Here's how the part is built. I have some questions about the finished solid (model axes, mm). A direction names the side the tool comes from. Round coordinates to 2 decimals unless told otherwise and drop trailing zeros. Write each loop counter-clockwise with the first axis right and the second up, starting at its lowest first coordinate (ties: lowest second). Pieces come first, ordered by that corner, then holes. Notation, with made-up numbers: (24.5, 30) -> (33.5, 30) arc R25 ccw to (33.5, 56) -> close; hole circle Ø4 at (16.5, -28). An arc over 180 degrees is marked (long way). Answer as CSV lines item,"result".
from build123d import *

# Parameters (mm, degrees)
F2_DEPTH  = 6.35
F3_DEPTH  = 25.4
F5_DEPTH  = 63.5
F6_W      = 35.5600007778
F6_H      = 6.6786579132
F7_DEPTH  = 25.4
F8_W      = 6.5081897405
F8_H      = 35.5600007778
F9_DEPTH  = 57.15
F10_W     = 35.5600007778
F10_H     = 6.35
F11_DEPTH = 19.05
F12_R     = 5.08
F13_R     = 5.08
F14_R     = 5.08
F15_R     = 5.08
F16_R     = 5.08


# Not quite as in the source:
# - two fillets or chamfers of one size are made in one step


with BuildPart() as f2:
    # F0 (on Top) → F2 (new body)
    with BuildSketch(Plane.XY):
        with BuildLine():
            ThreePointArc((-18.3481574059, -1.8204556262), (-18.2829820174, -0.6015784588), (-18.3481574059, 0.6172987085))
            Line((-18.3481574059, 0.6172987085), (-18.3481574059, -1.8204556262))
        make_face()
        with BuildLine():
            Line((-29.7129820174, 10.8284215412), (-64.0681574059, 10.8284215412))
            Line((-64.0681574059, 10.8284215412), (-64.0681574059, 5.8474093676))
            Line((-64.0681574059, 5.8474093676), (-65.235733552, 5.8474093676))
            Line((-65.235733552, 5.8474093676), (-65.235733552, -6.7013129592))
            Line((-65.235733552, -6.7013129592), (-64.0681574059, -6.7013129592))
            Line((-64.0681574059, -6.7013129592), (-64.0681574059, -12.0315784588))
            Line((-64.0681574059, -12.0315784588), (-60.0158534944, -12.0315784588))
            Line((-60.0158534944, -12.0315784588), (-60.0158534944, -14.5130921155))
            Line((-60.0158534944, -14.5130921155), (-49.2716534944, -14.5130921155))
            Line((-49.2716534944, -14.5130921155), (-49.2716534944, -12.0315784588))
            Line((-49.2716534944, -12.0315784588), (-29.7129820174, -12.0315784588))
            ThreePointArc((-29.7129820174, -12.0315784588), (-22.0738350108, -9.1038330429), (-18.3481574059, -1.8204556262))
            Line((-18.3481574059, -1.8204556262), (-18.3481574059, 0.6172987085))
            ThreePointArc((-18.3481574059, 0.6172987085), (-22.0738350108, 7.9006761252), (-29.7129820174, 10.8284215412))
        make_face()
    extrude(amount=-F2_DEPTH)

    # F1 (on Top) → F3 (join)
    with BuildSketch(Plane.XY):
        with BuildLine():
            Line((-42.9216531055, -18.3815788478), (-29.7129820174, -18.3815788478))
            ThreePointArc((-29.7129820174, -18.3815788478), (-17.6903920931, -13.7006526758), (-11.9981570169, -2.1225613757))
            Line((-11.9981570169, -2.1225613757), (-11.9981570169, 0.919404458))
            ThreePointArc((-11.9981570169, 0.919404458), (-17.6903920931, 12.4974957581), (-29.7129820174, 17.1784219301))
            Line((-29.7129820174, 17.1784219301), (-70.4181577948, 17.1784219301))
            Line((-70.4181577948, 17.1784219301), (-70.4181577948, 12.1974097565))
            Line((-70.4181577948, 12.1974097565), (-70.4181577948, -13.0513133481))
            Line((-70.4181577948, -13.0513133481), (-70.4181577948, -18.3815788478))
            Line((-70.4181577948, -18.3815788478), (-66.3658538833, -18.3815788478))
            Line((-66.3658538833, -18.3815788478), (-42.9216531055, -18.3815788478))
        make_face()
    extrude(amount=-F3_DEPTH)

    # F4 (on face) → F5 (join)
    with BuildSketch(Plane.XY):
        with BuildLine():
            Line((-42.9216538833, -18.3815788478), (-29.7129820174, -18.3815788478))
            ThreePointArc((-29.7129820174, -18.3815788478), (-17.6903920931, -13.7006526758), (-11.9981570169, -2.1225613757))
            Line((-11.9981570169, -2.1225613757), (-11.9981570169, 0.919404458))
            ThreePointArc((-11.9981570169, 0.919404458), (-17.6903920931, 12.4974957581), (-29.7129820174, 17.1784219301))
            Line((-29.7129820174, 17.1784219301), (-70.4181577948, 17.1784219301))
            Line((-70.4181577948, 17.1784219301), (-70.4181577948, 12.1974097565))
            Line((-70.4181577948, 12.1974097565), (-70.4181577948, -13.0513133481))
            Line((-70.4181577948, -13.0513133481), (-70.4181577948, -18.3815788478))
            Line((-70.4181577948, -18.3815788478), (-66.3658538833, -18.3815788478))
            Line((-66.3658538833, -18.3815788478), (-42.9216538833, -18.3815788478))
        make_face()
        with BuildLine():
            Line((-65.2357339409, 5.8474097565), (-64.0681577948, 5.8474097565))
            Line((-64.0681577948, 5.8474097565), (-64.0681577948, 10.8284219301))
            Line((-64.0681577948, 10.8284219301), (-29.7129820174, 10.8284219301))
            ThreePointArc((-29.7129820174, 10.8284219301), (-22.0738347431, 7.9006764075), (-18.3481570169, 0.6172987293))
            Line((-18.3481570169, 0.6172987293), (-18.3481570169, -1.820455647))
            ThreePointArc((-18.3481570169, -1.820455647), (-22.0738347431, -9.1038333252), (-29.7129820174, -12.0315788478))
            Line((-29.7129820174, -12.0315788478), (-49.2716531055, -12.0315788478))
            Line((-49.2716531055, -12.0315788478), (-49.2716531055, -14.5130925044))
            Line((-49.2716531055, -14.5130925044), (-60.0158538833, -14.5130925044))
            Line((-60.0158538833, -14.5130925044), (-60.0158538833, -12.0315788478))
            Line((-60.0158538833, -12.0315788478), (-64.0681577948, -12.0315788478))
            Line((-64.0681577948, -12.0315788478), (-64.0681577948, -6.7013133481))
            Line((-64.0681577948, -6.7013133481), (-65.2357339409, -6.7013133481))
            Line((-65.2357339409, -6.7013133481), (-65.2357339409, 5.8474097565))
        make_face(mode=Mode.SUBTRACT)
    extrude(amount=F5_DEPTH)

    # F6 (on face) → F7 (join)
    with BuildSketch(Plane(origin=(-70.4181577948, 0, 0), x_dir=(0, -1, 0), z_dir=(-1, 0, 0))):
        with Locations((0.6015784588, -22.0606710434)):
            Rectangle(F6_W, F6_H)
    extrude(amount=F7_DEPTH)

    # F8 (on face) → F9 (join)
    with BuildSketch(Plane.XY.offset(-18.7213420868)):
        with Locations((-92.5640629245, -0.6015784588)):
            Rectangle(F8_W, F8_H)
    extrude(amount=F9_DEPTH)

    # F10 (on face) → F11 (join)
    with BuildSketch(Plane.YZ.offset(-89.3099680543)):
        with Locations((-0.6015784588, 35.2536579132)):
            Rectangle(F10_W, F10_H)
    extrude(amount=F11_DEPTH)

    # F12
    f12_edges = [f2.edges().sort_by_distance(p)[0] for p in [
        (-95.818158, -0.601578, 38.428658),
    ]]
    fillet(f12_edges, radius=F12_R)

    # F13
    f13_edges = [f2.edges().sort_by_distance(p)[0] for p in [
        (-95.818158, -0.601578, -25.4),
    ]]
    fillet(f13_edges, radius=F13_R)

    # F14
    f14_edges = [f2.edges().sort_by_distance(p)[0] for p in [
        (-70.418158, -18.381579, 6.678658),
    ]]
    fillet(f14_edges, radius=F14_R)

    # F15
    f15_edges = [f2.edges().sort_by_distance(p)[0] for p in [
        (-70.418158, 17.178422, 6.678658),
    ]]
    fillet(f15_edges, radius=F15_R)

    # F16
    f16_edges = [f2.edges().sort_by_distance(p)[0] for p in [
        (-89.309968, 17.178422, 6.678658),
        (-89.309968, -18.381579, 6.678658),
    ]]
    fillet(f16_edges, radius=F16_R)


solid = f2.part
Item 1: Suppose I cut it at A-A, the plane z = 18. List the corners of the cut face in (x, y) for me, then the cut area to 3 significant figures.
Results found:
outline,"(-95.82, -18.38) -> (-94.39, -18.38) arc R5.08 ccw to (-89.31, -13.3) -> (-89.31, 12.1) arc R5.08 ccw to (-94.39, 17.18) -> (-95.82, 17.18) -> close; (-70.42, -13.3) arc R5.08 ccw to (-65.34, -18.38) -> (-29.71, -18.38) arc R17.78 ccw to (-12, -2.12) -> (-12, 0.92) arc R17.78 ccw to (-29.71, 17.18) -> (-65.34, 17.18) arc R5.08 ccw to (-70.42, 12.1) -> close; hole (-65.24, -6.7) -> (-64.07, -6.7) -> (-64.07, -12.03) -> (-60.02, -12.03) -> (-60.02, -14.51) -> (-49.27, -14.51) -> (-49.27, -12.03) -> (-29.71, -12.03) arc R11.43 ccw to (-18.35, -1.82) -> (-18.35, 0.62) arc R11.43 ccw to (-29.71, 10.83) -> (-64.07, 10.83) -> (-64.07, 5.85) -> (-65.24, 5.85) -> close"
area,"1,120 mm²"
Item 2: I need wall thicknesses on L1, parallel to Y at x = -55.5, z = 23; L2, parallel to Y at x = -45, z = 45; L3, parallel to Z at x = -60, y = -10.5. Which ranges of each line are inside material? Lowest first, please.
Results found:
L1,"y = -18.38 to -14.51, 10.83 to 17.18"
L2,"y = -18.38 to -12.03, 10.83 to 17.18"
L3,"z = -25.4 to 0"
Item 3: If we mould it in two halves opening along X, with no side actions, what happens to faces 1 (the flat face through (-70.418, 0, 6)), 2 (the flat face through (-11.998, -1, 18)), 3 (the flat face through (-42, 12, 63.5))? For each: pulls with the +X half, pulls with the -X half, needs draft (parallel to the pull), parting line crosses it, or undercut.
Results found:
face 1,"undercut"
face 2,"pulls with the +X half"
face 3,"needs draft"
Item 4: Suppose I cut it at D-D, the plane x = -54. List the corners of the cut face in (y, z) for me, then the cut area to 3 significant figures.
Results found:
outline,"(-18.38, -25.4) -> (17.18, -25.4) -> (17.18, 63.5) -> (10.83, 63.5) -> (10.83, 0) -> (-14.51, 0) -> (-14.51, 63.5) -> (-18.38, 63.5) -> close"
area,"1,550 mm²"
Item 5: Will these pins go through, and if not, where does the flat tip stop? pin 1 (4 mm diameter, centred on y = -11.5, z = 36.5, fed in from +X); pin 2 (20 mm diameter, centred on y = 6.5, z = 54, fed in from -X); pin 3 (2 mm diameter, centred on y = -14, z = 36.5, fed in from -X); pin 4 (10 mm diameter, centred on y = -6, z = 49, fed in from +X).
Results found:
pin 1,"stops at x = -14.32"
pin 2,"stops at x = -70.42"
pin 3,"stops at x = -95.34"
pin 4,"stops at x = -12"
Item 6: Suppose I cut it at B-B, the plane x = -87. List the corners of the cut face in (y, z) for me, then the cut area to 3 significant figures.
Results found:
outline,"(-18.38, -25.4) -> (17.18, -25.4) -> (17.18, -18.72) -> (-18.38, -18.72) -> close; (-18.38, 32.08) -> (17.18, 32.08) -> (17.18, 38.43) -> (-18.38, 38.43) -> close"
area,"463 mm²"
Item 7: Suppose I cut it at C-C, the plane z = -16. List the corners of the cut face in (x, y) for me.
Results found:
outline,"(-95.82, -18.38) -> (-94.39, -18.38) arc R5.08 ccw to (-89.31, -13.3) -> (-89.31, 12.1) arc R5.08 ccw to (-94.39, 17.18) -> (-95.82, 17.18) -> close; (-70.42, -13.3) arc R5.08 ccw to (-65.34, -18.38) -> (-29.71, -18.38) arc R17.78 ccw to (-12, -2.12) -> (-12, 0.92) arc R17.78 ccw to (-29.71, 17.18) -> (-65.34, 17.18) arc R5.08 ccw to (-70.42, 12.1) -> close"
Item 8: For faces 4 (the flat face through (-64.068, 8, 31)), 5 (the cylindrical face through (-17.555, 12.372, 18.428)), 6 (the flat face through (-70.418, 0, 51)), which set-ups out of +Z, -Z, +X, -X, +Y, -Y let a thin tool reach every point of the face, with its end or its side?
Results found:
face 4,"+Z"
face 5,"+Z, -Z, +X, +Y"
face 6,"+Z, -X, +Y, -Y"
